from build123d import *

# Parameters (mm, degrees)
SKETCH1_W               = 25.4
SKETCH1_H               = 25.4
SKETCH1_W_2             = 22.225
SKETCH1_H_2             = 22.225
EXTRUDE_THIN1_DEPTH     = 355.6
F_3_8_CLEARANCE_HOLE1_D = 9.8044


with BuildPart() as part:
    # Sketch1 → Extrude-Thin1 (new body)
    with BuildSketch(Plane(origin=(0, 0, 0), x_dir=(1, 0, 0), z_dir=(0, 1, 0))):
        Rectangle(SKETCH1_W, SKETCH1_H)
        Rectangle(SKETCH1_W_2, SKETCH1_H_2, mode=Mode.SUBTRACT)
    extrude(amount=EXTRUDE_THIN1_DEPTH)

    # 3/8 Clearance Hole1 (through all)
    with Locations(Plane(origin=(0, 0, -12.7), x_dir=(-1, 0, 0), z_dir=(0, 0, -1))):
        with Locations((0, 345.6), (0, 320.6), (0, 35), (0, 10)):
            Hole(F_3_8_CLEARANCE_HOLE1_D / 2)


solid = part.part
Build history of the part. All positions in model axes, mm. A direction names the side the tool comes from. Round coordinates to 2 decimals unless told otherwise and drop trailing zeros. Loops run counter-clockwise (first coordinate to the right, second up) from the corner with the lowest first, then second, coordinate; pieces in that order, holes last. Notation, with made-up numbers: (11.25, 44) -> (43.25, 44) arc R18 cw to (43.25, 70) -> close; hole circle Ø4 at (-27.5, 56). An arc over 180 degrees is marked (long way). One line per item, written item: value. Start each with the question number.
Q1. 3-axis set-ups, long thin cutter, end or side, ignore diameter. For faces 1 (the face through (0, 175, -11.112)), 2 (the face through (-1.063, 30.214, -11.895)): which of +Z, -Z, +X, -X, +Y, -Y reach the whole face in a straight line?
Q2. Cut at A-A on y = 165.5. List the corners of the cut face in (x, z).
Q3. Cut at B-B on z = 2.75. List the corners of the cut face in (x, y), plus the area to 3 significant figures.
Q4. Cut at C-C on y = 35. List the corners of the cut face in (x, z).
Q5. Probe line 1 along Y through (x, z) = (0, -12.1); line 2 along X through (y, z) = (265, -4.25). List the from-to ranges inside material, lowest first.
Q6. Cut at D-D on x = 0. Count the separate pieces of the cut face and the enclosed holes in it, plus the area to 3 significant figures.
Q7. Drop a flat-ended pin along its axis: pin 1 Ø8 at (x, z) = (-3.5, 3.5) entering from -Y. Give the stop position or say it passes through.
Q8. Two-plate mould, pull along Z, no slides. Class faces 3 (the face through (-11.112, 175, 0)), 4 (the face through (11.112, 175, 0)), 5 (the face through (0, 175, -12.7)), 6 (the face through (-0.64, 350.46, -11.9)): released by +Z, released by -Z, zero draft, split by the parting line, or undercut.
Computed:
1. face 1: +Y, -Y
1. face 2: +Z, -Z
2. outline: (-12.7, -12.7) -> (12.7, -12.7) -> (12.7, 12.7) -> (-12.7, 12.7) -> close; hole (-11.11, -11.11) -> (11.11, -11.11) -> (11.11, 11.11) -> (-11.11, 11.11) -> close
3. outline: (-12.7, 0) -> (-11.11, 0) -> (-11.11, 355.6) -> (-12.7, 355.6) -> close; (11.11, 0) -> (12.7, 0) -> (12.7, 355.6) -> (11.11, 355.6) -> close
3. area: 1,130 mm²
4. outline: (-12.7, -12.7) -> (-4.9, -12.7) -> (-4.9, -11.11) -> (-11.11, -11.11) -> (-11.11, 11.11) -> (-4.9, 11.11) -> (-4.9, 12.7) -> (-12.7, 12.7) -> close; (4.9, -12.7) -> (12.7, -12.7) -> (12.7, 12.7) -> (4.9, 12.7) -> (4.9, 11.11) -> (11.11, 11.11) -> (11.11, -11.11) -> (4.9, -11.11) -> close
5. line 1: 0 to 5.1, 14.9 to 30.1, 39.9 to 315.7, 325.5 to 340.7, 350.5 to 355.6
5. line 2: -12.7 to -11.11, 11.11 to 12.7
6. separate pieces: 10
6. enclosed holes: 0
6. area: 1,000 mm²
7. pin 1: through
8. face 3: undercut
8. face 4: undercut
8. face 5: released by -Z
8. face 6: zero draft
